Geometry check sheet. Reference: the model listing, model coordinates, mm. A direction names the side the tool comes from. Round coordinates to 2 decimals unless told otherwise and drop trailing zeros. Loops run counter-clockwise (first coordinate to the right, second up) from the corner with the lowest first, then second, coordinate; pieces in that order, holes last. Notation, with made-up numbers: M 82.5,7 L 127.5,7 A13 cw 127.5,28 Z; hole C -34,36.5 d8. An arc over 180 degrees is marked long. Write item = value, one per line.
from build123d import *

# Parameters (mm, degrees)
F0_R     = 3.75
F1_DEPTH = 4
F3_DEPTH = 5
F4_DEPTH = 5


with BuildPart() as f1:
    # F0 (on Top) → F1 (new body)
    with BuildSketch(Plane.XY):
        Circle(F0_R)
    extrude(amount=F1_DEPTH)

    # F2 (on face) → F3 (cut, symmetric)
    with BuildSketch(Plane.XY.offset(4)):
        with BuildLine():
            ThreePointArc((3, -1.25), (3.186887196, -0.6373774392), (3.25, 0))
            ThreePointArc((3.25, 0), (3.186887196, 0.6373774392), (3, 1.25))
            ThreePointArc((3, 1.25), (0, 3.25), (-3, 1.25))
            ThreePointArc((-3, 1.25), (-3.25, 0), (-3, -1.25))
            ThreePointArc((-3, -1.25), (0, -3.25), (3, -1.25))
        make_face()
    extrude(amount=F3_DEPTH, both=True, mode=Mode.SUBTRACT)

    # F2 (on face) → F4 (join)
    with BuildSketch(Plane.XY.offset(4)):
        with BuildLine():
            ThreePointArc((-3, 1.25), (0, 3.25), (3, 1.25))
            Line((3, 1.25), (3, 2.25))
            ThreePointArc((3, 2.25), (1.6770509831, 3.3541019662), (0, 3.75))
            ThreePointArc((0, 3.75), (-1.6770509831, 3.3541019662), (-3, 2.25))
            Line((-3, 2.25), (-3, 1.25))
        make_face()
        with BuildLine():
            Line((3, -2.25), (3, -1.25))
            ThreePointArc((3, -1.25), (0, -3.25), (-3, -1.25))
            Line((-3, -1.25), (-3, -2.25))
            ThreePointArc((-3, -2.25), (-1.6770509831, -3.3541019662), (0, -3.75))
            ThreePointArc((0, -3.75), (1.6770509831, -3.3541019662), (3, -2.25))
        make_face()
    extrude(amount=F4_DEPTH)


solid = f1.part
(1) Sectioned sample at B-B on z = 7. Record the cut outline in (x, y).
Result set:
outline = M -3,-2.25 A3.75 ccw 3,-2.25 L 3,-1.25 A3.25 cw -3,-1.25 Z; M -3,1.25 A3.25 cw 3,1.25 L 3,2.25 A3.75 ccw -3,2.25 Z
(2) Sectioned sample at D-D on z = 0.75. Record the cut outline in (x, y).
Result set:
outline = C 0,0 d7.5; hole C 0,0 d6.5
(3) Material ranges on line 1 along X through (y, z) = (0, 3); line 2 along X through (y, z) = (3, 7.25), recorded low to high. Write a range as from..to.
Result set:
line_1 = -3.75..-3.25, 3.25..3.75
line_2 = -2.25..-1.25, 1.25..2.25
(4) Depth check by flat-ended pin: pin 1 Ø0.8 at (x, y) = (3.5, -0.5) entering from +Z; pin 2 Ø1.5 at (x, z) = (-1.5, 8) entering from -Y; pin 3 Ø0.5 at (y, z) = (-1.5, 6) entering from -X. Enter the tip coordinate at first touch or a pass-through.
Result set:
pin_1 = 4
pin_2 = -3.67
pin_3 = -3
(5) Sectioned sample at C-C on x = 0.75. Record the cut outline in (y, z).
Result set:
outline = M -3.67,0 L -3.16,0 L -3.16,9 L -3.67,9 Z; M 3.16,0 L 3.67,0 L 3.67,9 L 3.16,9 Z
(6) Sectioned sample at A-A on y = 0. Record the cut outline in (x, z).
Result set:
outline = M -3.75,0 L -3.25,0 L -3.25,4 L -3.75,4 Z; M 3.25,0 L 3.75,0 L 3.75,4 L 3.25,4 Z
(7) Tool access check on faces 1 (the flat face through (-3, -2, 6)), 2 (the flat face through (0, 3.4, 0)), 3 (the flat face through (3, 2, 6)). Record the directions out of +Z, -Z, +X, -X, +Y, -Y that give a thin tool (end or side, any length) a straight path to the whole face; none if there is none.
Result set:
face_1 = +Z, -X, +Y, -Y
face_2 = -Z, +X, -X, +Y, -Y
face_3 = +Z, +X, +Y, -Y
